Autodesk Inventor part; units mm, degrees
ref_plane "Work Plane1" through (-14.5, -35, 0) normal (0, -1, 0) x (1, 0, 0)
ref_plane "Work Plane4" through (-14.5, -35, 0) normal (-1, 0, 0) x (0, 0, 1)
ref_plane "YZ Plane" through (0, 0, 0) normal (1, 0, 0) x (0, 1, 0)
ref_plane "Work Plane1" through (-14.5, -35, 0) normal (0, -1, 0) x (1, 0, 0)
sketch "Sketch2" plane through (-14.5, -35, 0) normal (0, -1, 0) x (1, 0, 0)
  line L0 (4.3469, 0) -> (4.3469, 20)
  line L1 (7.596, 20) -> (7.4184, 20)
  line L2 (4.3469, 20) -> (7.596, 20)
  arc A0 (7.596, 20) -> (29, 8.6937) centre (18.17, 14.1045) ccw
  line L3 (4.3469, 0) -> (18.3998, 0)
  arc A1 (18.3998, 0) -> (29, 8.6937) centre (18.9461, 10.1431) ccw
  point P0 (14.5, 0)
  point P1 (5, 0)
  point P2 (18.2531, 1.9984)
extrude "Extrusion1" add sketch "Sketch2" against normal blind 10
ref_plane "Work Plane4" through (-14.5, -35, 0) normal (-1, 0, 0) x (0, 0, 1)
sketch "Sketch3" plane through (-14.5, -35, 0) normal (-1, 0, 0) x (0, 0, 1)
  line L0 (20, 0) -> (20, 70)
  line L1 (0, 0) -> (0, 21)
  line L2 (20, 70) -> (0, 70)
  line L3 (0, 70) -> (0, 0)
  line L4 (0, 0) -> (20, 0)
  line L5 (20, 0) -> (20, 70)
  point P0 (0, 35)
extrude "Extrusion2" add sketch "Sketch3" against normal blind 5.5
mirror "Mirror3" about plane through (0, 0, 0) normal (0, 1, 0) of "Extrusion1"
sketch "Sketch4" plane through (-9, -35, 0) normal (1, 0, 0) x (0, 0, -1)
  line L0 (-20, 10) -> (-1.9981, 10)
  line L1 (-12.7438, 10) -> (-12.7438, 60)
  line L2 (0, 60) -> (-20, 60)
  line L3 (-12.7438, 35) -> (-17.7089, 35)
  circle A0 centre (-12.7438, 35) radius 1.5
  point P0 (0, 35)
  point P1 (-8.6937, 10)
  dimension "d4" = 3
extrude "Extrusion3" cut sketch "Sketch4" against normal blind 10.375
sketch "Sketch5" plane through (-14.5, -35, 0) normal (-1, 0, 0) x (0, 0, 1)
  line L0 (20, 70) -> (0, 70)
  line L1 (0, 0) -> (20, 0)
  line L2 (20, 70) -> (0, 70)
  line L3 (0, 70) -> (0, 0)
  line L4 (0, 0) -> (20, 0)
  line L5 (20, 0) -> (20, 70)
  point P0 (0, 35)
extrude "Extrusion4" cut sketch "Sketch5" against normal blind 2
sketch "Sketch7" plane through (-14.5, -35, 0) normal (0, -1, 0) x (1, 0, 0)
  line L0 (7.596, 20) -> (2, 20)
  line L1 (2, 20) -> (2, 0)
  line L2 (2, 20) -> (2, 0)
  line L3 (2, 0) -> (19.4924, 0)
  arc A0 (18.3998, 0) -> (29, 8.6937) centre (18.9461, 10.1431) ccw
  line L4 (5.5, 20) -> (7.596, 20)
  arc A1 (7.596, 20) -> (29, 8.6937) centre (18.17, 14.1045) ccw
  arc A2 (7.596, 20) -> (29, 8.6937) centre (18.17, 14.1045) ccw
  arc A3 (19.4924, 0) -> (29, 8.6937) centre (18.9461, 10.1431) ccw
  line L5 (2, 20) -> (7.596, 20)
  point P0 (14.5, 0)
extrude "Extrusion5" cut sketch "Sketch7" against normal blind 1 contours A1 A0 L3 L1 L0
sketch "Sketch8" plane through (-12.5, 35, 0) normal (0, 1, 0) x (1, 0, 0)
  line L0 (3.5, -20) -> (5.596, -20)
  line L1 (0, 0) -> (0, -20)
  line L2 (5.596, -20) -> (0, -20)
  line L3 (0, -20) -> (0, 0)
  arc A0 (27, -8.6937) -> (16.3998, 0) centre (16.9461, -10.1431) ccw
  line L4 (0, 0) -> (16.3998, 0)
  arc A1 (27, -8.6937) -> (5.596, -20) centre (16.17, -14.1045) ccw
  arc A2 (27, -8.6937) -> (5.596, -20) centre (16.17, -14.1045) ccw
  arc A3 (27, -8.6937) -> (16.3998, 0) centre (16.9461, -10.1431) ccw
  point P0 (12.5, 0)
extrude "Extrusion6" cut sketch "Sketch8" against normal blind 1
properties part number "Speed Champ"
For this review, take the finished solid that the model builds, in its own axes (mm). A direction names the side the tool comes from. Round coordinates to 2 decimals unless told otherwise and drop trailing zeros. Write each loop counter-clockwise with the first axis right and the second up, starting at its lowest first coordinate (ties: lowest second). Pieces come first, ordered by that corner, then holes. Notation, with made-up numbers: (-34.5, 46) - (-21.5, 46) arc R18 ccw to (-21.5, 55) - close; hole circle Ø1 at (6, 20). An arc over 180 degrees is marked (long way). Use a Markdown table: item, result.
Q1. We need section A-A (y = 0). Give the boundary of the cut face in (x, z), plus the area to 3 significant figures.
Derived:
| item | result |
|---|---|
| outline | (-12.5, 0) - (-9, 0) - (-9, 11.24) - (-12.5, 11.24) - close; (-12.5, 14.24) - (-9, 14.24) - (-9, 20) - (-12.5, 20) - close |
| area | 59.5 mm2 |
Q2. Machinability: for faces 5 (the flat face through (-9, 0, 10)), 6 (the flat face through (-7, 34, 8)), which of the approach directions +Z, -Z, +X, -X, +Y, -Y give a long, thin tool a straight path to every point of the face, cutting with its end or side? Answer none if there is none.
Derived:
| item | result |
|---|---|
| face 5 | +Z, -Z, +X |
| face 6 | +Z, -Z, +X, -X, +Y |
Q3. Clearance check with flat-ended pins moving along their axes: pin 1 (6 mm diameter, centred on y = 4, z = 12.5, fed in from +X); pin 2 (0.5 mm diameter, centred on x = 4.5, y = -34.5, fed in from +Z). State where each tip first meets the part, or that it passes through.
Derived:
| item | result |
|---|---|
| pin 1 | stops at x = -9 |
| pin 2 | stops at z = 0 |
Q4. We need section C-C (z = 5). Give the boundary of the cut face in (x, y).
Derived:
| item | result |
|---|---|
| outline | (-12.5, -34) - (-4.31, -34) - (-4.31, -25) - (-9, -25) - (-9, 25) - (-4.31, 25) - (-4.31, 34) - (-12.5, 34) - close; (11.65, -34) - (13.21, -34) - (13.21, -25) - (11.65, -25) - close; (11.65, 25) - (13.21, 25) - (13.21, 34) - (11.65, 34) - close |
Q5. The part is to be moulded in two halves that separate along X. For faces 1 (the flat face through (-10, 0, 0)), 2 (the cylindrical face through (-2.222, -29.563, 3.529)), 3 (the flat face through (-12.5, 0, 10)), 4 (the cylindrical face through (-1.744, 29.563, 3.276)), say which applies: pulls with the +X half, pulls with the -X half, needs draft (parallel to the pull), parting line crosses it, or undercut.
Derived:
| item | result |
|---|---|
| face 1 | needs draft |
| face 2 | undercut |
| face 3 | pulls with the -X half |
| face 4 | undercut |
Q6. Wall thickness on line 1 along Z through (x, y) = (-11.6, 0); line 2 along Y through (x, z) = (-7, 8); line 3 along X through (y, z) = (-28, 13.5): over which ranges is each line inside the solid? List them lowest first.
Derived:
| item | result |
|---|---|
| line 1 | z = 0 to 11.24, 14.24 to 20 |
| line 2 | y = -34 to -25, 25 to 34 |
| line 3 | x = -12.5 to -8.42 |
Q7. We need section B-B (x = -0.5). Give the boundary of the cut face in (y, z), plus the area to 3 significant figures.
Derived:
| item | result |
|---|---|
| outline | (-34, 0) - (-25, 0) - (-25, 2.74) - (-34, 2.74) - close; (25, 0) - (34, 0) - (34, 2.74) - (25, 2.74) - close |
| area | 49.3 mm2 |
